Geometry check sheet. Reference: the model listing, model coordinates, mm. A direction names the side the tool comes from. Give positions to 0.01 mm unless a question says otherwise; leave off trailing zeros. Order: outer loops, then holes, each group sorted by start corner. A loop starts at its lowest first (then second) coordinate and runs counter-clockwise, first axis right, second up.
```python
from build123d import *

# Parameters (mm, degrees)
SKETCH1_W            = 40
SKETCH1_H            = 17
SKETCH1_R            = 3.6
SKETCH1_R_2          = 1.6
BOSS_EXTRUDE1_DEPTH  = 4
SKETCH2_W            = 7
SKETCH2_H            = 3
BOSS_EXTRUDE2_DEPTH  = 20
SKETCH3_R            = 1.597664911
SKETCH3_R_2          = 1.6
CUT_EXTRUDE1_DEPTH   = 20
BOSS_EXTRUDE3_DEPTH  = 2
FILLET1_R            = 10
FILLET1_OF_MIRROR1_R = 10
SKETCH5_R            = 3
CUT_EXTRUDE2_DEPTH   = 2


with BuildPart() as part:
    # Sketch1 → Boss-Extrude1 (new body)
    with BuildSketch(Plane.XY):
        Rectangle(SKETCH1_W, SKETCH1_H)
        Circle(SKETCH1_R, mode=Mode.SUBTRACT)
        with Locations((8.5, 0)):
            Circle(SKETCH1_R_2, mode=Mode.SUBTRACT)
        with Locations(Location((-8.5, 0, 0), (0, 0, 180))):
            Circle(SKETCH1_R_2, mode=Mode.SUBTRACT)
    extrude(amount=BOSS_EXTRUDE1_DEPTH)

    # Sketch2 → Boss-Extrude2 (add)
    with BuildSketch(Plane(origin=(0, 0, 0), x_dir=(-1, 0, 0), z_dir=(0, 0, -1))):
        with Locations((16.5, -7)):
            Rectangle(SKETCH2_W, SKETCH2_H)
    boss_extrude2 = extrude(amount=BOSS_EXTRUDE2_DEPTH)

    # Sketch3 → Cut-Extrude1 (cut)
    with BuildSketch(Plane(origin=(0, -5.5, 0), x_dir=(1, 0, 0), z_dir=(0, 1, 0))):
        with Locations(Location((-16.5, 4, 0), (0, 0, 180))):
            Circle(SKETCH3_R)
        with Locations(Location((-16.5, 16, 0), (0, 0, 180))):
            Circle(SKETCH3_R_2)
    cut_extrude1 = extrude(amount=-CUT_EXTRUDE1_DEPTH, mode=Mode.SUBTRACT)

    # Sketch4 → Boss-Extrude3 (add)
    with BuildSketch(Plane.ZY.offset(20)):
        Polygon((0, 3.19845738), (-11.998610201, -5.5), (-11.998610201, -8.5), (4, -8.5), (4, 3.19845738), align=None)
    boss_extrude3 = extrude(amount=BOSS_EXTRUDE3_DEPTH)

    # Fillet1
    # the kernel refuses this fillet: 10 mm, written as the material it takes off along each edge
    with BuildSketch(Plane(origin=(-22, 9.5, -11.998610201), x_dir=(0, 0, 1), z_dir=(0, -1, 0))) as fillet1_piece_1:
        with BuildLine():
            CenterArc((6, -10), FILLET1_R, 90, 36.869897646)
            Line((0, -2), (-0.12, -1.84))
            ThreePointArc((-0.12, -1.84), (-0.2, -1), (-0.2, 0))
            Line((-0.2, 0), (0, 0.2))
            Line((0, 0.2), (6, 0.2))
            Line((6, 0.2), (6, 0))
        make_face()
    extrude(amount=33, mode=Mode.SUBTRACT)
    with BuildSketch(Plane(origin=(-22, 3.19845738, 19), x_dir=(1, 0, 0), z_dir=(0, 0, -1))) as fillet1_piece_2:
        with BuildLine():
            CenterArc((10, 6), FILLET1_R, 180, 36.869897646)
            Line((0, 6), (-0.2, 6))
            Line((-0.2, 6), (-0.2, 0))
            Line((-0.2, 0), (0, -0.2))
            ThreePointArc((0, -0.2), (1, -0.2), (1.84, -0.12))
            Line((1.84, -0.12), (2, 0))
        make_face()
    extrude(amount=34, mode=Mode.SUBTRACT)

    # Mirror1: Boss-Extrude2, Cut-Extrude1, Boss-Extrude3 across plane
    add(boss_extrude2.mirror(Plane(origin=(0, 0, 0), x_dir=(0, 0, 1), z_dir=(1, 0, 0))))
    add(cut_extrude1.mirror(Plane(origin=(0, 0, 0), x_dir=(0, 0, 1), z_dir=(1, 0, 0))), mode=Mode.SUBTRACT)
    add(boss_extrude3.mirror(Plane(origin=(0, 0, 0), x_dir=(0, 0, 1), z_dir=(1, 0, 0))))

    # Fillet1 of Mirror1
    # the kernel refuses this fillet: 10 mm, written as the material it takes off along each edge
    with BuildSketch(Plane(origin=(22, 9.5, -11.998610201), x_dir=(-1, 0, 0), z_dir=(0, -1, 0))) as fillet1_of_mirror1_piece_1:
        with BuildLine():
            CenterArc((10, -6), FILLET1_OF_MIRROR1_R, 143.130102354, 36.869897646)
            Line((0, -6), (-0.2, -6))
            Line((-0.2, -6), (-0.2, 0))
            Line((-0.2, 0), (0, 0.2))
            ThreePointArc((0, 0.2), (1, 0.2), (1.84, 0.12))
            Line((1.84, 0.12), (2, 0))
        make_face()
    extrude(amount=33, mode=Mode.SUBTRACT)
    with BuildSketch(Plane(origin=(22, 3.19845738, 19), x_dir=(-1, 0, 0), z_dir=(0, 0, -1))) as fillet1_of_mirror1_piece_2:
        with BuildLine():
            CenterArc((10, -6), FILLET1_OF_MIRROR1_R, 143.130102354, 36.869897646)
            Line((0, -6), (-0.2, -6))
            Line((-0.2, -6), (-0.2, 0))
            Line((-0.2, 0), (0, 0.2))
            ThreePointArc((0, 0.2), (1, 0.2), (1.84, 0.12))
            Line((1.84, 0.12), (2, 0))
        make_face()
    extrude(amount=34, mode=Mode.SUBTRACT)

    # Sketch5 → Cut-Extrude2 (cut)
    with BuildSketch(Plane.XY.offset(4)):
        with Locations((-8.5, 0)):
            Circle(SKETCH5_R)
        with Locations((8.5, 0)):
            Circle(SKETCH5_R)
    extrude(amount=-CUT_EXTRUDE2_DEPTH, mode=Mode.SUBTRACT)


solid = part.part
```
Q1. Cross-section at B-B, the plane x = 16.5. Record the boundary of the cut face in (y, z).
Q2. Cross-section at D-D, the plane x = 0. Record the boundary of the cut face in (y, z), and give its area (3 significant figures).
Q3. Access from +Z, -Z, +X, -X, +Y, -Y to the whole of each face (thin tool, end or side, straight path). Record for faces 1 (the face through (11.27, -1.15, 3.01)), 2 (the face through (0, 4, 0)), 3 (the face through (-13, -7, -10)).
Q4. Cross-section at A-A, the plane z = -16. Record the boundary of the cut face in (x, y).
Q5. Thickness scan on L1, parallel to Z at x = 16.5, y = -7.35; L2, parallel to Y at x = 8.5, z = 3.25; L3, parallel to Z at x = 7, y = 3.75. Record the ranges inside material, lowest first.
Q6. Cross-section at C-C, the plane y = -6. Record the boundary of the cut face in (x, z).
Q7. Gauge pin test, flat ends, axial feed: P1, Ø6, axis at x = -11, y = -3.5, coming from the -Z side; P2, Ø2.5, axis at y = -7, z = -14.5, coming from the -X side; P3, Ø4, axis at x = 16.5, z = -16, coming from the +Y side; P4, Ø6, axis at y = 0.5, z = -7.5, coming from the +X side. Record the tip position at first contact, or that the pin passes through.
Q8. Release check for a two-part mould opening along Y. For faces 4 (the face through (20, -3, -3)), 5 (the face through (-5.73, -1.15, 3.01)), 6 (the face through (16, -5.5, -10)) record: pulls with the +Y half, pulls with the -Y half, needs draft (parallel to the pull), parting line crosses it, or undercut.
Answers follow:
1. outline: (-8.5, -20) - (-5.5, -20) - (-5.5, -17.6) - (-8.5, -17.6) - close; (-8.5, -14.4) - (-5.5, -14.4) - (-5.5, -5.6) - (-8.5, -5.6) - close; (-8.5, -2.4) - (-5.5, -2.4) - (-5.5, 0) - (8.5, 0) - (8.5, 4) - (-8.5, 4) - close
2. outline: (-8.5, 0) - (-3.6, 0) - (-3.6, 4) - (-8.5, 4) - close; (3.6, 0) - (8.5, 0) - (8.5, 4) - (3.6, 4) - close
2. area: 39.2 mm2
3. face 1: +Z
3. face 2: -Z, +Y
3. face 3: -Z, +Y, -Y
4. outline: (-20, -8.5) - (-18.1, -8.5) - (-18.1, -5.5) - (-20, -5.5) - close; (-14.9, -8.5) - (-13, -8.5) - (-13, -5.5) - (-14.9, -5.5) - close; (13, -8.5) - (14.9, -8.5) - (14.9, -5.5) - (13, -5.5) - close; (18.1, -8.5) - (20, -8.5) - (20, -5.5) - (18.1, -5.5) - close
5. L1: z = -20 to -17.6, -14.4 to -5.6, -2.4 to 4
5. L2: y = -8.5 to -3, 3 to 8.5
5. L3: z = 0 to 4
6. outline: (-22, -6) arc R10 ccw to (-20, -12) - (-20, -20) - (-13, -20) - (-13, 0) - (13, 0) - (13, -20) - (20, -20) - (20, -12) arc R10 ccw to (22, -6) - (22, 4) - (-22, 4) - close; hole circle Ø3.2 at (-16.5, -16); hole circle Ø3.2 at (-16.5, -4); hole circle Ø3.2 at (16.5, -16); hole circle Ø3.2 at (16.5, -4)
7. P1: stops at z = -20
7. P2: stops at x = -20
7. P3: stops at y = -5.5
7. P4: stops at x = 21.99
8. face 4: needs draft
8. face 5: undercut
8. face 6: pulls with the +Y half
